Check sheet for the modelled part. Datum: model origin and axes. Units: mm. Coordinates: 2 decimals unless noted, no trailing zeros. Loops run counter-clockwise (first coordinate to the right, second up) from the corner with the lowest first, then second, coordinate; pieces in that order, holes last. Notation, with made-up numbers: (1.5, 76.25) -> (43.5, 76.25) arc R16 ccw to (43.5, 88.25) -> close; hole circle Ø4 at (7.25, -10.5). An arc over 180 degrees is marked (long way). Use one line per item in the form item = value.
from build123d import *

# Parameters (mm, degrees)
SKETCH1_W           = 5.013785632
SKETCH1_H           = 9.926537354
SKETCH1_R           = 2.1
BOSS_EXTRUDE2_DEPTH = 1.2
FILLET1_R           = 2


with BuildPart() as part:
    # Sketch1 → Boss-Extrude2 (new body)
    with BuildSketch(Plane.XY):
        Rectangle(SKETCH1_W, SKETCH1_H)
        with Locations((0, 2.378079684)):
            Circle(SKETCH1_R, mode=Mode.SUBTRACT)
        with Locations((0, -2.52414688)):
            Circle(SKETCH1_R, mode=Mode.SUBTRACT)
    extrude(amount=BOSS_EXTRUDE2_DEPTH)

    # Fillet1
    fillet1_edges = [part.edges().sort_by_distance(p)[0] for p in [
        (2.506892816, -4.963268677, 0.6),
        (-2.506892816, -4.963268677, 0.6),
        (-2.506892816, 4.963268677, 0.6),
        (2.506892816, 4.963268677, 0.6),
    ]]
    fillet(fillet1_edges, radius=FILLET1_R)


solid = part.part
(1) Section check A-A, the plane x = 0. Record the boundary of the cut face in (y, z), plus the area to 3 significant figures.
Established:
outline = (-4.96, 0) -> (-4.62, 0) -> (-4.62, 1.2) -> (-4.96, 1.2) -> close; (-0.42, 0) -> (0.28, 0) -> (0.28, 1.2) -> (-0.42, 1.2) -> close; (4.48, 0) -> (4.96, 0) -> (4.96, 1.2) -> (4.48, 1.2) -> close
area = 1.83 mm²
(2) Go/stop test with a flat-tipped pin: P1, Ø2.5, axis at x = 0, y = 2.38, coming from the +Z side. Record where the tip stops, or that it passes through.
Established:
P1 = through
(3) Section check D-D, the plane y = -3.5. Record the boundary of the cut face in (x, z), plus the area to 3 significant figures.
Established:
outline = (-2.43, 0) -> (-1.86, 0) -> (-1.86, 1.2) -> (-2.43, 1.2) -> close; (1.86, 0) -> (2.43, 0) -> (2.43, 1.2) -> (1.86, 1.2) -> close
area = 1.38 mm²
(4) Section check B-B, the plane y = 1.25. Record the boundary of the cut face in (x, z).
Established:
outline = (-2.51, 0) -> (-1.77, 0) -> (-1.77, 1.2) -> (-2.51, 1.2) -> close; (1.77, 0) -> (2.51, 0) -> (2.51, 1.2) -> (1.77, 1.2) -> close
(5) Section check C-C, the plane z = 0.75. Record the boundary of the cut face in (x, y), plus the area to 3 significant figures.
Established:
outline = (-2.51, -2.96) arc R2 ccw to (-0.51, -4.96) -> (0.51, -4.96) arc R2 ccw to (2.51, -2.96) -> (2.51, 2.96) arc R2 ccw to (0.51, 4.96) -> (-0.51, 4.96) arc R2 ccw to (-2.51, 2.96) -> close; hole circle Ø4.2 at (0, -2.52); hole circle Ø4.2 at (0, 2.38)
area = 18.6 mm²
(6) Mould release check, pull along X, two halves, no side actions. Record for faces 1 (the flat face through (-2.507, 0, 1)), 2 (the cylindrical face through (-0.46, 0.33, 0.59)), 3 (the flat face through (0, 4.963, 1)), 4 (the cylindrical face through (1.9, -4.4, 0.6)): +X half, -X half, draft (parallel to the pull), parting line (faces both ways), or undercut.
Established:
face_1 = -X half
face_2 = undercut
face_3 = draft
face_4 = +X half
(7) Scan lines: line 1 along Y through (x, z) = (0, 0.6); line 2 along Y through (x, z) = (-1.8, 0.75); line 3 along X through (y, z) = (2.5, 0.1). Record each from-to range of solid material in increasing order.
Established:
line_1 = -4.96 to -4.62, -0.42 to 0.28, 4.48 to 4.96
line_2 = -4.49 to -3.61, -1.44 to 1.3, 3.46 to 4.49
line_3 = -2.51 to -2.1, 2.1 to 2.51
